Here's the drawing with two shaded views (mm, measured from the low corner). I have some questions. Round coordinates to 2 decimals unless told otherwise and drop trailing zeros. Order: outer loops, then holes, each group sorted by start corner. A loop starts at its lowest first (then second) coordinate and runs counter-clockwise, first axis right, second up.
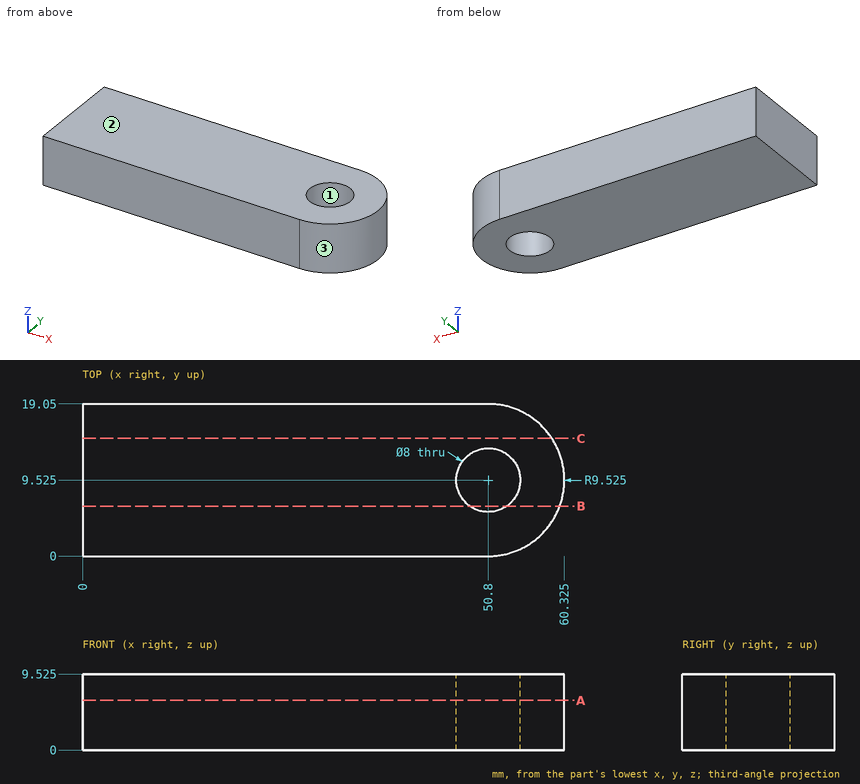
Q1. Imagine slicing it at A-A, the plane z = 6.25. Please give me the cut outline in (x, y) (3 decimals).
Q2. For P1, Ø8, axis at x = 41.5, y = 2.5, coming from the -Z side, with a flat end and sliding along its axis, tell me the tip position at first contact or that it passes through.
Q3. We'd pull the mould along Y, two halves only. Please class the marked faces 1, 2 and 3: released by +Y, released by -Y, zero draft, split by the parting line, or undercut.
Q4. I need wall thicknesses on L1, parallel to X at y = 9.25, z = 2; L2, parallel to X at y = 11, z = 4.5; L3, parallel to Y at x = 54, z = 5.25 (3 decimals). Which ranges of each line are inside material? Lowest first, please.
Q5. Imagine slicing it at C-C, the plane y = 14.75. Please give me the cut outline in (x, z) (3 decimals), then the cut area to 3 significant figures.
Q6. Imagine slicing it at B-B, the plane y = 6.25. Please give me the cut outline in (x, z) (3 decimals), then the cut area to 3 significant figures.
Filled in:
1. outline: (0, 0) - (50.8, 0) arc R9.525 ccw to (50.8, 19.05) - (0, 19.05) - close; hole circle Ø8 at (50.8, 9.525)
2. P1: stops at z = 0
3. face 1: undercut
3. face 2: zero draft
3. face 3: split by the parting line
4. L1: x = 0 to 46.81, 54.79 to 60.32
4. L2: x = 0 to 47.08, 54.52 to 60.21
4. L3: y = 0.554 to 7.125, 11.925 to 18.496
5. outline: (0, 0) - (58.764, 0) - (58.764, 9.525) - (0, 9.525) - close
5. area: 560 mm2
6. outline: (0, 0) - (48.503, 0) - (48.503, 9.525) - (0, 9.525) - close; (53.097, 0) - (59.744, 0) - (59.744, 9.525) - (53.097, 9.525) - close
6. area: 525 mm2
